The listing builds one solid part. Answer for the finished solid, in the listing's coordinates (mm). A direction names the side the tool comes from. Coordinates: 2 decimals unless noted, no trailing zeros. Write each loop counter-clockwise with the first axis right and the second up, starting at its lowest first coordinate (ties: lowest second). Pieces come first, ordered by that corner, then holes.
(1) Given P1, Ø4, axis at x = 72.5, y = -10.5, coming from the +Z side, flat-ended and moving along its own axis, determine where the tip first touches the part or whether it passes through.
(2) The part is cut by section B-B on y = -85. Determine the outline of the cut face in (x, z), plus the area to 3 significant figures.
(3) The part is cut by section C-C on x = 126.5. Determine the outline of the cut face in (y, z), plus the area to 3 significant figures.
(4) Straight lines are drawn through the part: line 1 (Y direction, x = -60, z = 32); line 2 (X direction, y = -6, z = 36); line 3 (X direction, y = 14.5, z = 42). For each, find the intervals that lie inside material, in ascending order.
(5) Which of the six approach directions +Z, -Z, +X, -X, +Y, -Y give full straight-line access (tool end or side, diameter ignored) to faces 4 (the flat face through (-2, -100, 38)), 5 (the flat face through (275, -4, 20))?
(6) For a pull along Y with two mould halves and no side action, classify faces 1 (the flat face through (-275, -4, 20)), 2 (the flat face through (-150, -1, 38)), 3 (the flat face through (-4, 275, 20)) as +Y half, -Y half, draft (parallel to the pull), parting line (faces both ways), or undercut.
(7) The part is cut by section A-A on z = 33. Determine the outline of the cut face in (x, y), plus the area to 3 significant figures.
from build123d import *

# Parameters (mm, degrees)
F0_W         = 550
F0_H         = 550
F1_DEPTH     = 50
F2_R         = 10
F3_T1_DEPTH  = 65
F3_S5_W      = 10
F3_S5_H      = 10
F3_T6_DEPTH  = 10
F3_S11_W     = 10
F3_S11_H     = 10
F3_T12_DEPTH = 10
F3_S17_W     = 10
F3_S17_H     = 10
F3_T18_DEPTH = 10
F3_S23_W     = 10
F3_S23_H     = 10
F3_T24_DEPTH = 10
F4_W         = 300
F4_H         = 200
F5_DEPTH     = 25


# Not quite as in the source:
# - a fillet or chamfer that OpenCascade refuses, or shapes differently, is made with other operations: its cross-section is extruded or revolved along the edge and cut away or added


with BuildPart() as f1:
    # F0 (on Top) → F1 (new body)
    with BuildSketch(Plane.XY):
        Rectangle(F0_W, F0_H)
    extrude(amount=F1_DEPTH)

    # F2
    f2_edges = [f1.edges().sort_by_distance(p)[0] for p in [
        (0, -275, 50),
        (275, 0, 50),
        (0, 275, 50),
        (-275, 0, 50),
    ]]
    fillet(f2_edges, radius=F2_R)

    # F3: fillet of radius 10 on 4 edges, made by hand

    # F3_s2 → F3_t1 (cut)
    with BuildSketch(Plane.XY.offset(-25)):
        with BuildLine():
            ThreePointArc((275, -265), (272.0710678119, -272.0710678119), (265, -275))
            Line((265, -275), (275, -275))
            Line((275, -275), (275, -265))
        make_face()
        with BuildLine():
            ThreePointArc((-265, -275), (-272.0710678119, -272.0710678119), (-275, -265))
            Line((-275, -265), (-275, -275))
            Line((-275, -275), (-265, -275))
        make_face()
        with BuildLine():
            ThreePointArc((-265, 275), (-272.0710678119, 272.0710678119), (-275, 265))
            Line((-275, 265), (-275, 275))
            Line((-275, 275), (-265, 275))
        make_face()
        with BuildLine():
            ThreePointArc((275, 265), (272.0710678119, 272.0710678119), (265, 275))
            Line((265, 275), (275, 275))
            Line((275, 275), (275, 265))
        make_face()
    extrude(amount=F3_T1_DEPTH, mode=Mode.SUBTRACT)


with BuildPart() as f3_tool4:
    # F3_s5 → F3_t6 (new body)
    with BuildSketch(Plane.YZ.offset(265)):
        with Locations((270, 45)):
            Rectangle(F3_S5_W, F3_S5_H)
    extrude(amount=F3_T6_DEPTH)

    # F3_s7 → F3_t8 (revolve, cut)
    with BuildSketch(Plane(origin=(265, 265, 40), x_dir=(0, -0.7071067812, -0.7071067812), z_dir=(0, -0.7071067812, 0.7071067812))):
        with BuildLine():
            ThreePointArc((0, -10), (10, 0), (0, 10))
            Line((0, 10), (0, -10))
        make_face()
    revolve(axis=Axis((265, 265, 40), (1, 0, 0)), mode=Mode.SUBTRACT)


with BuildPart() as f1_1:
    add(f1.part)

    # F3_t3: cut F3_tool4
    add(f3_tool4.part, mode=Mode.SUBTRACT)


with BuildPart() as f3_tool10:
    # F3_s11 → F3_t12 (new body)
    with BuildSketch(Plane.XZ.offset(-265)):
        with Locations((-270, 45)):
            Rectangle(F3_S11_W, F3_S11_H)
    extrude(amount=-F3_T12_DEPTH)

    # F3_s13 → F3_t14 (revolve, cut)
    with BuildSketch(Plane(origin=(-265, 265, 40), x_dir=(0.7071067812, 0, -0.7071067812), z_dir=(0.7071067812, 0, 0.7071067812))):
        with BuildLine():
            ThreePointArc((0, -10), (10, 0), (0, 10))
            Line((0, 10), (0, -10))
        make_face()
    revolve(axis=Axis((-265, 265, 40), (0, 1, 0)), mode=Mode.SUBTRACT)


with BuildPart() as f1_2:
    add(f1_1.part)

    # F3_t9: cut F3_tool10
    add(f3_tool10.part, mode=Mode.SUBTRACT)


with BuildPart() as f3_tool16:
    # F3_s17 → F3_t18 (new body)
    with BuildSketch(Plane.XZ.offset(265)):
        with Locations((-270, 45)):
            Rectangle(F3_S17_W, F3_S17_H)
    extrude(amount=F3_T18_DEPTH)

    # F3_s19 → F3_t20 (revolve, cut)
    with BuildSketch(Plane(origin=(-265, -265, 40), x_dir=(0.7071067812, 0, -0.7071067812), z_dir=(-0.7071067812, 0, -0.7071067812))):
        with BuildLine():
            ThreePointArc((0, -10), (10, 0), (0, 10))
            Line((0, 10), (0, -10))
        make_face()
    revolve(axis=Axis((-265, -265, 40), (0, -1, 0)), mode=Mode.SUBTRACT)


with BuildPart() as f1_3:
    add(f1_2.part)

    # F3_t15: cut F3_tool16
    add(f3_tool16.part, mode=Mode.SUBTRACT)


with BuildPart() as f3_tool22:
    # F3_s23 → F3_t24 (new body)
    with BuildSketch(Plane.YZ.offset(265)):
        with Locations((-270, 45)):
            Rectangle(F3_S23_W, F3_S23_H)
    extrude(amount=F3_T24_DEPTH)

    # F3_s25 → F3_t26 (revolve, cut)
    with BuildSketch(Plane(origin=(265, -265, 40), x_dir=(0, 0.7071067812, -0.7071067812), z_dir=(0, -0.7071067812, -0.7071067812))):
        with BuildLine():
            ThreePointArc((0, -10), (10, 0), (0, 10))
            Line((0, 10), (0, -10))
        make_face()
    revolve(axis=Axis((265, -265, 40), (1, 0, 0)), mode=Mode.SUBTRACT)


with BuildPart() as f1_4:
    add(f1_3.part)

    # F3_t21: cut F3_tool22
    add(f3_tool22.part, mode=Mode.SUBTRACT)

    # F4 (on face) → F5 (cut)
    with BuildSketch(Plane.XY.offset(50)):
        Rectangle(F4_W, F4_H)
    extrude(amount=-F5_DEPTH, mode=Mode.SUBTRACT)


solid = f1_4.part
Model answer:
1. P1: stops at z = 25
2. outline: (-275, 0) - (275, 0) - (275, 40) arc R10 ccw to (265, 50) - (150, 50) - (150, 25) - (-150, 25) - (-150, 50) - (-265, 50) arc R10 ccw to (-275, 40) - close
2. area: 20,000 mm2
3. outline: (-275, 0) - (275, 0) - (275, 40) arc R10 ccw to (265, 50) - (100, 50) - (100, 25) - (-100, 25) - (-100, 50) - (-265, 50) arc R10 ccw to (-275, 40) - close
3. area: 22,500 mm2
4. line 1: y = -275 to -100, 100 to 275
4. line 2: x = -275 to -150, 150 to 275
4. line 3: x = -274.8 to -150, 150 to 274.8
5. face 4: +Z
5. face 5: +Z, -Z, +X, +Y, -Y
6. face 1: draft
6. face 2: undercut
6. face 3: +Y half
7. outline: (-275, -265) arc R10 ccw to (-265, -275) - (265, -275) arc R10 ccw to (275, -265) - (275, 265) arc R10 ccw to (265, 275) - (-265, 275) arc R10 ccw to (-275, 265) - close; hole (-150, -100) - (150, -100) - (150, 100) - (-150, 100) - close
7. area: 242,000 mm2
